Part model, mm, in its own coordinate system. Face numbers are marked on the shaded views. A direction names the side the tool comes from. Coordinates: 2 decimals unless noted, no trailing zeros. Write each loop counter-clockwise with the first axis right and the second up, starting at its lowest first coordinate (ties: lowest second). Pieces come first, ordered by that corner, then holes. Notation, with made-up numbers: (39.25, 61.5) - (87.25, 61.5) arc R15 ccw to (87.25, 88.5) - close; hole circle Ø4 at (-14, 13.5). An arc over 180 degrees is marked (long way). Use a Markdown table: item, result.
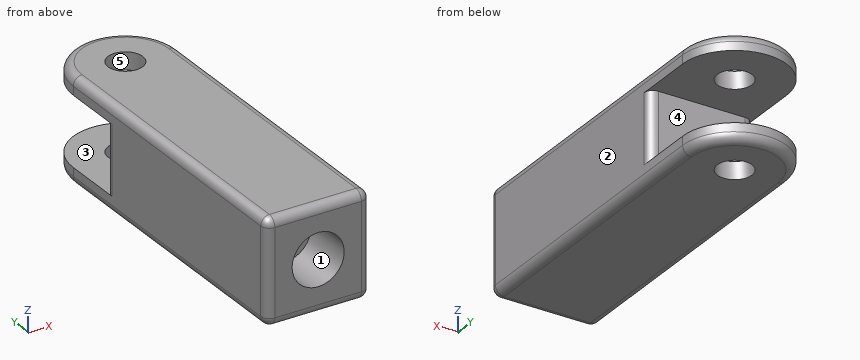
```python
from build123d import *

# Parameters (mm, degrees)
SKETCH_1_W          = 60
SKETCH_1_H          = 60
EXTRUDE_1_DEPTH     = 150
SKETCH_2_R          = 15
CUT_EXTRUDE_1_DEPTH = 30
SKETCH_3_R          = 10
EXTRUDE_2_DEPTH     = 60
SKETCH_4_W          = 40
SKETCH_4_H          = 60
CUT_EXTRUDE_2_DEPTH = 61
FILLET_1_R          = 5


with BuildPart() as part:
    # 草圖1 → 填料-伸長1 (new body)
    with BuildSketch(Plane(origin=(0, 0, 0), x_dir=(1, 0, 0), z_dir=(0, 1, 0))):
        Rectangle(SKETCH_1_W, SKETCH_1_H)
    extrude(amount=EXTRUDE_1_DEPTH)

    # 草圖2 → 除料-伸長1 (cut)
    with BuildSketch(Plane.XZ):
        Circle(SKETCH_2_R)
    extrude(amount=-CUT_EXTRUDE_1_DEPTH, mode=Mode.SUBTRACT)

    # 草圖3 → 填料-伸長2 (add)
    with BuildSketch(Plane.XY.offset(30)):
        with BuildLine():
            Line((-30, 150), (-30, 175))
            ThreePointArc((-30, 175), (0, 205), (30, 175))
            Line((30, 175), (30, 150))
            Line((30, 150), (-30, 150))
        make_face()
        with Locations((0, 175)):
            Circle(SKETCH_3_R, mode=Mode.SUBTRACT)
    extrude(amount=-EXTRUDE_2_DEPTH)

    # 草圖4 → 除料-伸長2 (cut, through all)
    with BuildSketch(Plane.ZY.offset(30)):
        with Locations((0, 175)):
            Rectangle(SKETCH_4_W, SKETCH_4_H)
    extrude(amount=-CUT_EXTRUDE_2_DEPTH, mode=Mode.SUBTRACT)

    # 圓角1
    fillet_1_edges = [part.edges().sort_by_distance(p)[0] for p in [
        (0, 205, 30),
        (0, 205, -30),
        (-30, 145, 0),
        (30, 145, 0),
        (0, 0, 30),
        (-30, 0, 0),
        (0, 0, -30),
        (30, 0, 0),
        (30, 87.5, 30),
        (-30, 87.5, 30),
        (-30, 87.5, -30),
        (30, 87.5, -30),
    ]]
    fillet(fillet_1_edges, radius=FILLET_1_R)


solid = part.part
```
Item 1: Band-saw the part on C-C, the plane z = 0. Give the cut face in (x, y), then the cut area to 3 significant figures.
From the geometry:
| item | result |
|---|---|
| outline | (-30, 5) arc R5 ccw to (-25, 0) - (-15, 0) - (-15, 30) - (15, 30) - (15, 0) - (25, 0) arc R5 ccw to (30, 5) - (30, 140) arc R5 ccw to (25, 145) - (-25, 145) arc R5 ccw to (-30, 140) - close |
| area | 7,780 mm^2 |
Item 2: Band-saw the part on B-B, the plane x = 0. Give the cut face in (y, z).
From the geometry:
| item | result |
|---|---|
| outline | (0, -25) arc R5 ccw to (5, -30) - (165, -30) - (165, -20) - (145, -20) - (145, 20) - (165, 20) - (165, 30) - (5, 30) arc R5 ccw to (0, 25) - (0, 15) - (30, 15) - (30, -15) - (0, -15) - close; (185, -30) - (200, -30) arc R5 ccw to (205, -25) - (205, -20) - (185, -20) - close; (185, 20) - (205, 20) - (205, 25) arc R5 ccw to (200, 30) - (185, 30) - close |
Item 3: Drop a flat-ended pin along its axis: P1, Ø8, axis at x = 15.5, z = -14, coming from the +Y side. Give the stop position or say it passes through.
From the geometry:
| item | result |
|---|---|
| P1 | y = 145 |
Item 4: Two-plate mould, pull along Y, no slides. Class the marked faces 3, 4 and 5: pulls with the +Y half, pulls with the -Y half, needs draft (parallel to the pull), parting line crosses it, or undercut.
From the geometry:
| item | result |
|---|---|
| face 3 | needs draft |
| face 4 | pulls with the +Y half |
| face 5 | undercut |
Item 5: Band-saw the part on A-A, the plane y = 25. Give the cut face in (x, z).
From the geometry:
| item | result |
|---|---|
| outline | (-30, -25) arc R5 ccw to (-25, -30) - (25, -30) arc R5 ccw to (30, -25) - (30, 25) arc R5 ccw to (25, 30) - (-25, 30) arc R5 ccw to (-30, 25) - close; hole circle Ø30 at (0, 0) |
Item 6: Drill centre lines: probe 1 along Y at (x, z) = (0, -24); probe 2 along Z at (x, y) = (0, 13.75); probe 3 along Y at (x, z) = (25, -11). Where is each one in solid material? Low to high.
From the geometry:
| item | result |
|---|---|
| probe 1 | 0 to 165, 185 to 205 |
| probe 2 | -30 to -15, 15 to 30 |
| probe 3 | 0 to 145 |
Item 7: Which spindle directions (+Z, -Z, +X, -X, +Y, -Y) get a long thin tool onto all of the face, cutting with end or side? Do the marked faces 1 and 2. Say none if no direction does.
From the geometry:
| item | result |
|---|---|
| face 1 | -Y |
| face 2 | +Z, -Z, +X, +Y, -Y |
